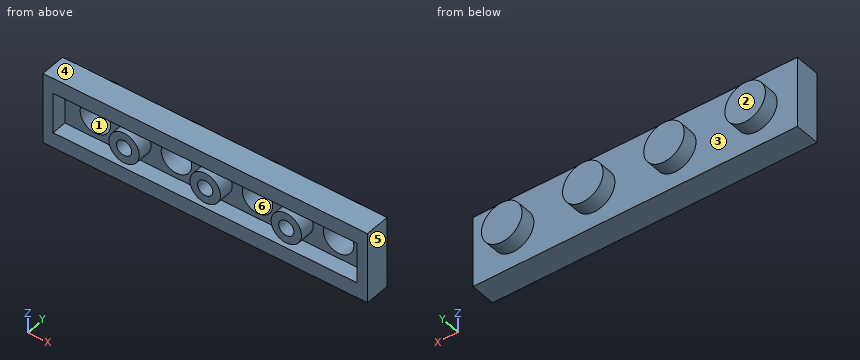
from build123d import *

# Parameters (mm, degrees)
SKETCH1_W           = 40.64
SKETCH1_H           = 3.175
BOSS_EXTRUDE1_DEPTH = 4.445
SKETCH2_R           = 2.54
BOSS_EXTRUDE2_DEPTH = 1.905
SKETCH3_W           = 38.1
SKETCH3_H           = 5.08
CUT_EXTRUDE1_DEPTH  = 1.905
SKETCH4_R           = 1.905
CUT_EXTRUDE2_DEPTH  = 2.54
SKETCH5_R           = 1.905
SKETCH5_R_2         = 0.9525
BOSS_EXTRUDE3_DEPTH = 1.905


with BuildPart() as part:
    # Sketch1 → Boss-Extrude1 (new body, symmetric)
    with BuildSketch(Plane.XY):
        with Locations((0, -1.5875)):
            Rectangle(SKETCH1_W, SKETCH1_H)
    extrude(amount=BOSS_EXTRUDE1_DEPTH, both=True)

    # Sketch2 → Boss-Extrude2 (add)
    with BuildSketch(Plane(origin=(0, 0, 0), x_dir=(1, 0, 0), z_dir=(0, 1, 0))):
        with Locations((-15.24, 0)):
            Circle(SKETCH2_R)
        with Locations((-5.08, 0)):
            Circle(SKETCH2_R)
        with Locations((5.08, 0)):
            Circle(SKETCH2_R)
        with Locations((15.24, 0)):
            Circle(SKETCH2_R)
    extrude(amount=BOSS_EXTRUDE2_DEPTH)

    # Sketch3 → Cut-Extrude1 (cut)
    with BuildSketch(Plane.XZ.offset(3.175)):
        Rectangle(SKETCH3_W, SKETCH3_H)
    extrude(amount=-CUT_EXTRUDE1_DEPTH, mode=Mode.SUBTRACT)

    # Sketch4 → Cut-Extrude2 (cut)
    with BuildSketch(Plane.XZ.offset(1.27)):
        with Locations((-15.24, 0)):
            Circle(SKETCH4_R)
        with Locations((-5.08, 0)):
            Circle(SKETCH4_R)
        with Locations((5.08, 0)):
            Circle(SKETCH4_R)
        with Locations((15.24, 0)):
            Circle(SKETCH4_R)
    extrude(amount=-CUT_EXTRUDE2_DEPTH, mode=Mode.SUBTRACT)

    # Sketch5 → Boss-Extrude3 (add)
    with BuildSketch(Plane.XZ.offset(1.27)):
        with Locations((-10.16, 0)):
            Circle(SKETCH5_R)
        with Locations((-10.16, 0)):
            Circle(SKETCH5_R_2, mode=Mode.SUBTRACT)
        with Locations((10.16, 0)):
            Circle(SKETCH5_R)
        with Locations((10.16, 0)):
            Circle(SKETCH5_R_2, mode=Mode.SUBTRACT)
        Circle(SKETCH5_R)
        Circle(SKETCH5_R_2, mode=Mode.SUBTRACT)
    extrude(amount=BOSS_EXTRUDE3_DEPTH)


solid = part.part
Here's how the part is built. I have some questions about the finished solid (model axes, mm). Face numbers are marked on the shaded views. A direction names the side the tool comes from. Round coordinates to 2 decimals unless told otherwise and drop trailing zeros. Write each loop counter-clockwise with the first axis right and the second up, starting at its lowest first coordinate (ties: lowest second). Pieces come first, ordered by that corner, then holes.
1. Suppose I cut it at C-C (z = 3.75). List the corners of the cut face in (x, y) for me (3 decimals).
2. Suppose I cut it at D-D (x = 15.24). List the corners of the cut face in (y, z) for me (3 decimals).
3. I need wall thicknesses on L1, parallel to Z at x = -9, y = -1.85 (3 decimals); L2, parallel to X at y = -1.9, z = 2; L3, parallel to Z at x = -15.24, y = 0.35 (3 decimals). Which ranges of each line are inside material? Lowest first, please.
4. Suppose I cut it at A-A (y = -2). State how many separate pieces and enclosed holes the cut face has, and give its area (3 significant figures).
5. For the marked faces 1, 2 and 3, which set-ups out of +Z, -Z, +X, -X, +Y, -Y let a thin tool reach every point of the face, with its end or its side?
6. Suppose I cut it at B-B (x = 0). List the corners of the cut face in (y, z) for me (1 decimal).
7. If we mould it in two halves opening along X, with no side actions, what happens to the marked faces 4, 5 and 6? For each: released by +X, released by -X, zero draft, split by the parting line, or undercut.
8. Will these pins go through, and if not, where does the flat tip stop? pin 1 Ø2.5 at (x, z) = (0, 0) entering from +Y; pin 2 Ø4 at (x, z) = (-5.5, 0.5) entering from -Y.
Answer sheet:
1. outline: (-20.32, -3.175) - (20.32, -3.175) - (20.32, 0) - (-20.32, 0) - close
2. outline: (-3.175, -4.445) - (0, -4.445) - (0, -2.54) - (1.905, -2.54) - (1.905, 2.54) - (0, 2.54) - (0, 4.445) - (-3.175, 4.445) - (-3.175, 2.54) - (-1.27, 2.54) - (-1.27, 1.905) - (1.27, 1.905) - (1.27, -1.905) - (-1.27, -1.905) - (-1.27, -2.54) - (-3.175, -2.54) - close
3. L1: z = -4.445 to -2.54, -1.511 to 1.511, 2.54 to 4.445
3. L2: x = -20.32 to -19.05, 19.05 to 20.32
3. L3: z = -2.54 to -1.905, 1.905 to 2.54
4. separate pieces: 4
4. enclosed holes: 4
4. area: 193 mm2
5. face 1: -Y
5. face 2: +Z, -Z, +X, -X, +Y
5. face 3: +Y
6. outline: (-3.2, -4.4) - (0, -4.4) - (0, 4.4) - (-3.2, 4.4) - (-3.2, 2.5) - (-1.3, 2.5) - (-1.3, 1.9) - (-3.2, 1.9) - (-3.2, 1) - (-1.3, 1) - (-1.3, -1) - (-3.2, -1) - (-3.2, -1.9) - (-1.3, -1.9) - (-1.3, -2.5) - (-3.2, -2.5) - close
7. face 4: zero draft
7. face 5: released by +X
7. face 6: undercut
8. pin 1: stops at y = 0
8. pin 2: stops at y = -1.27
